from build123d import *

# Parameters (mm, degrees)
SKETCH1_W               = 65
SKETCH1_H               = 30
BOSS_EXTRUDE1_DEPTH     = 14
SKETCH2_W               = 48
SKETCH2_H               = 32
CUT_EXTRUDE1_DEPTH      = 8
CUT_EXTRUDE2_DEPTH      = 55.046276467
CUT_EXTRUDE2_DEPTH_BACK = 55.046276467
SKETCH3_R               = 5.1


with BuildPart() as part:
    # Sketch1 → Boss-Extrude1 (new, symmetric)
    with BuildSketch(Plane.XY):
        with Locations((17.5, 0)):
            Rectangle(SKETCH1_W, SKETCH1_H)
    extrude(amount=BOSS_EXTRUDE1_DEPTH, both=True)

    # Sketch2 → Cut-Extrude1 (cut, symmetric)
    with BuildSketch(Plane.XY):
        with Locations((8, 0)):
            Rectangle(SKETCH2_W, SKETCH2_H)
    extrude(amount=CUT_EXTRUDE1_DEPTH, both=True, mode=Mode.SUBTRACT)

    # Sketch3 → Cut-Extrude2 (cut, two sides: drawn at the far end of the back side and taken through both)
    with BuildSketch(Plane.XY.offset(-CUT_EXTRUDE2_DEPTH_BACK)):
        Circle(SKETCH3_R)
    extrude(amount=CUT_EXTRUDE2_DEPTH + CUT_EXTRUDE2_DEPTH_BACK, mode=Mode.SUBTRACT)


solid = part.part
Here's how the part is built. I have some questions about the finished solid (model axes, mm). A direction names the side the tool comes from. Coordinates: 2 decimals unless noted, no trailing zeros. Write each loop counter-clockwise with the first axis right and the second up, starting at its lowest first coordinate (ties: lowest second). Pieces come first, ordered by that corner, then holes.
1) Thinking about a two-plate mould opening in Y: for faces 3 (the face through (-15, 0, 11)), 4 (the face through (2.4, -4.5, -11)), 5 (the face through (24, 15, 10)), which applies, +Y half, -Y half, draft (parallel to the pull), parting line (faces both ways), or undercut?
Filled in:
face 3: draft
face 4: undercut
face 5: +Y half
2) If we section it at B-B (y = 0): List the corners of the cut face in (x, z) for me, plus the area to 3 significant figures.
Filled in:
outline: (-15, -14) - (-5.1, -14) - (-5.1, -8) - (-15, -8) - close; (-15, 8) - (-5.1, 8) - (-5.1, 14) - (-15, 14) - close; (5.1, -14) - (50, -14) - (50, 14) - (5.1, 14) - (5.1, 8) - (32, 8) - (32, -8) - (5.1, -8) - close
area: 946 mm2
3) I'm going to push flat-ended pins straight in: pin 1 (10 mm diameter, centred on y = 9, z = -2, fed in from -X); pin 2 (3 mm diameter, centred on x = 4, z = -5, fed in from -Y). Where does each tip first touch, or does it pass through?
Filled in:
pin 1: stops at x = 32
pin 2: passes through
4) If we section it at C-C (x = 25.5): List the corners of the cut face in (y, z) for me, plus the area to 3 significant figures.
Filled in:
outline: (-15, -14) - (15, -14) - (15, -8) - (-15, -8) - close; (-15, 8) - (15, 8) - (15, 14) - (-15, 14) - close
area: 360 mm2
5) Which directions (+Z, -Z, +X, -X, +Y, -Y) give clear straight access to the entire face, cutting with the end or side of a thin tool? Please do faces 1 (the face through (17, 0, 14)), 2 (the face through (8, 0, -8)).
Filled in:
face 1: +Z, +X, -X, +Y, -Y
face 2: -X, +Y, -Y
6) If we section it at D-D (z = 8.75): List the corners of the cut face in (x, y) for me, plus the area to 3 significant figures.
Filled in:
outline: (-15, -15) - (50, -15) - (50, 15) - (-15, 15) - close; hole circle Ø10.2 at (0, 0)
area: 1,870 mm2
7) If we section it at A-A (x = 0): List the corners of the cut face in (y, z) for me.
Filled in:
outline: (-15, -14) - (-5.1, -14) - (-5.1, -8) - (-15, -8) - close; (-15, 8) - (-5.1, 8) - (-5.1, 14) - (-15, 14) - close; (5.1, -14) - (15, -14) - (15, -8) - (5.1, -8) - close; (5.1, 8) - (15, 8) - (15, 14) - (5.1, 14) - close
8) If I drill on line 1 (X direction, y = 0, z = -10.55); line 2 (Z direction, x = 28, y = -2.75); line 3 (Y direction, x = 0, z = -9.5), over which ranges is the centre line in solid material (lowest first)?
Filled in:
line 1: x = -15 to -5.1, 5.1 to 50
line 2: z = -14 to -8, 8 to 14
line 3: y = -15 to -5.1, 5.1 to 15
